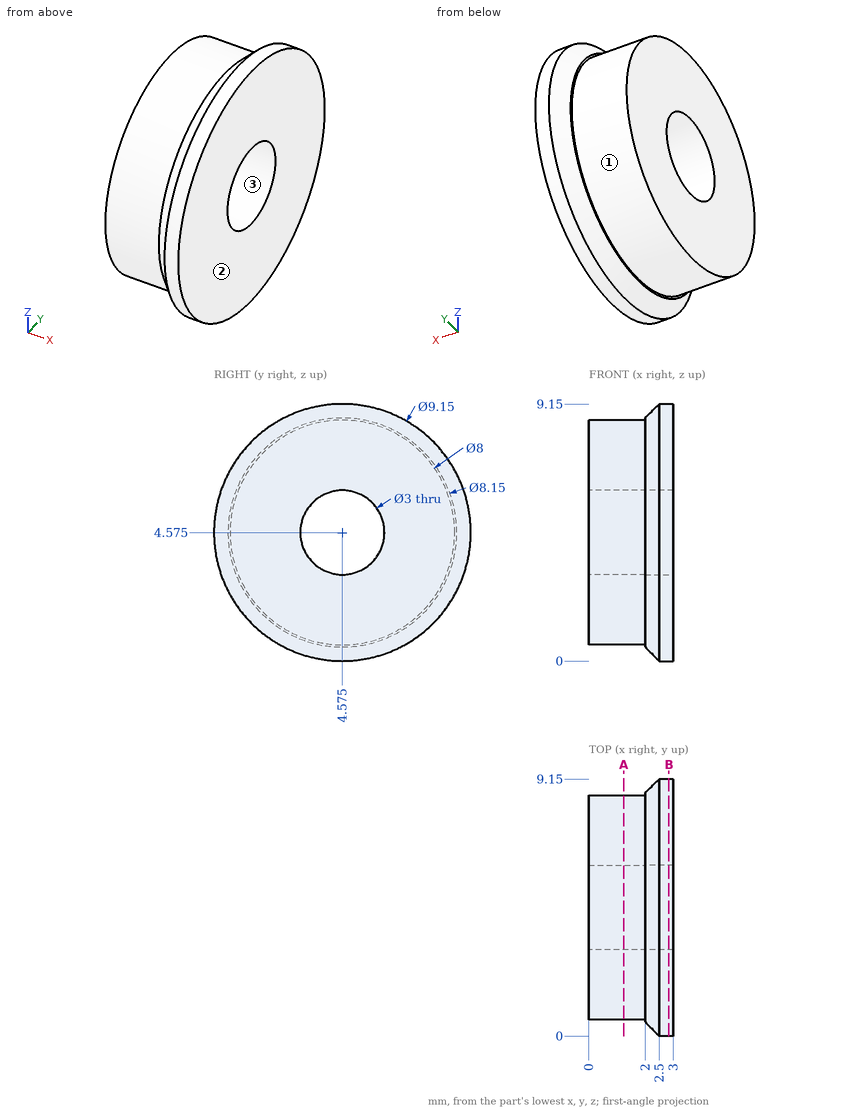
Design review of the part shown in the three views and the two pictorial views. Dimensions are in mm from the part's minimum x, y and z. Give positions to 0.01 mm unless a question says otherwise; leave off trailing zeros. Loops run counter-clockwise (first coordinate to the right, second up) from the corner with the lowest first, then second, coordinate; pieces in that order, holes last. Notation, with made-up numbers: (84.5, 37.25) -> (119.5, 37.25) arc R15 ccw to (119.5, 41.25) -> close; hole circle Ø5 at (-13.75, 28.5). An arc over 180 degrees is marked (long way). Write each question's results on one line, items separated by ' | '.
Q1. Wall thickness on L1, parallel to Y at x = 0.15, z = 4.5; L2, parallel to Z at x = 0.2, y = 3.25; L3, parallel to Z at x = 2.35, y = 5.25: over which ranges is each line inside the solid? List them lowest first.
Reply:
L1: y = 0.58 to 3.08, 6.07 to 8.57 | L2: z = 0.8 to 3.87, 5.28 to 8.35 | L3: z = 0.2 to 3.24, 5.91 to 8.95
Q2. Take a section at B-B, the plane x = 2.85. Write out the cut boundary in (y, z) (3 decimals), plus the area to 3 significant figures.
Reply:
outline: circle Ø9.15 at (4.575, 4.575); hole circle Ø3 at (4.575, 4.575) | area: 58.7 mm²
Q3. The part is to be moulded in two halves that separate along Y. For the marked faces 1, 2 and 3, say which applies: +Y half, -Y half, draft (parallel to the pull), parting line (faces both ways), or undercut.
Reply:
face 1: parting line | face 2: draft | face 3: undercut
Q4. Take a section at A-A, the plane x = 1.25. Write out the cut boundary in (y, z) (3 decimals), plus the area to 3 significant figures.
Reply:
outline: circle Ø8 at (4.575, 4.575); hole circle Ø3 at (4.575, 4.575) | area: 43.2 mm²
Q5. For pin 1 Ø2.5 at (y, z) = (4.575, 4.575) entering from +X; pin 2 Ø1 at (x, z) = (0.5, 3) entering from +Y; pin 3 Ø1 at (y, z) = (4, 1.5) entering from -X, all flat-tipped, find the tip position at first contact; note any pin that passes through.
Reply:
pin 1: passes through | pin 2: stops at y = 8.43 | pin 3: stops at x = 0
